Geometry: final body of the model. Coordinates: model frame, mm. Round coordinates to 2 decimals unless told otherwise and drop trailing zeros. Loops run counter-clockwise (first coordinate to the right, second up) from the corner with the lowest first, then second, coordinate; pieces in that order, holes last. Notation, with made-up numbers: M 54.5,39 L 96.5,39 A22 cw 96.5,76 Z; hole C 54.5,-26.75 d5. An arc over 180 degrees is marked long. Answer as a JSON object with one key per item and string values.
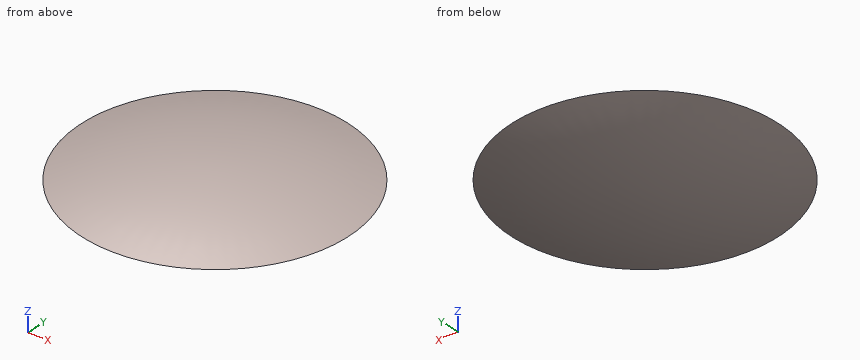
```python
from build123d import *

# Parameters (mm, degrees)
SCALE1_SCALE = 0.75


with BuildPart() as part:
    # Sketch1 → Revolve1 (revolve)
    with BuildSketch(Plane(origin=(0, 0, 0), x_dir=(0, 0, -1), z_dir=(1, 0, 0))):
        with BuildLine():
            Line((0, 0), (0, 22.5))
            ThreePointArc((0, 22.5), (2.640052345, 11.387396334), (3.527205849, 0))
            Line((3.527205849, 0), (0, 0))
        make_face()
    revolve1 = revolve(axis=Axis((0, 0, 34.553258587), (0, 0, -1)))

    # Mirror1: Revolve1 across plane
    add(revolve1.mirror(Plane.XY))


with BuildPart() as part_1:
    # Scale1: scaled about (0, 0, 0)
    add(part.part.scale(SCALE1_SCALE))


solid = part_1.part
```
1) First-contact query: pin 1 (10 mm diameter, centred on x = 4.5, y = 5, fed in from +Z); pin 2 (10 mm diameter, centred on x = -1.5, y = 12.5, fed in from +Z); pin 3 (5 mm diameter, centred on x = 4.5, y = 12.5, fed in from -Z). Flat tips, straight axial feed; report the tip coordinate or a pass-through.
Geometry results:
{"pin 1": "z = 2.62", "pin 2": "z = 2.12", "pin 3": "z = -1.58"}
2) Cut plane A-A on x = -10. Return the cut outline in (y, z).
Geometry results:
{"outline": "M -13.59,0 A54.23 ccw 13.59,0 A54.23 ccw Z"}
3) Cut plane B-B on y = -14. Return the cut outline in (x, z).
Geometry results:
{"outline": "M -9.42,0 A53.34 ccw 9.42,0 A53.34 ccw Z"}
4) Cut plane C-C on z = 1.2. Return the cut outline in (x, y).
Geometry results:
{"outline": "C 0,0 d25.09"}
5) Line query: probe 1 along Z at (x, y) = (10.5, -9.5); probe 2 along Z at (x, y) = (-8, 2). Output: solid intervals per line, ascending.
Geometry results:
{"probe 1": "-0.8 to 0.8", "probe 2": "-2.03 to 2.03"}
